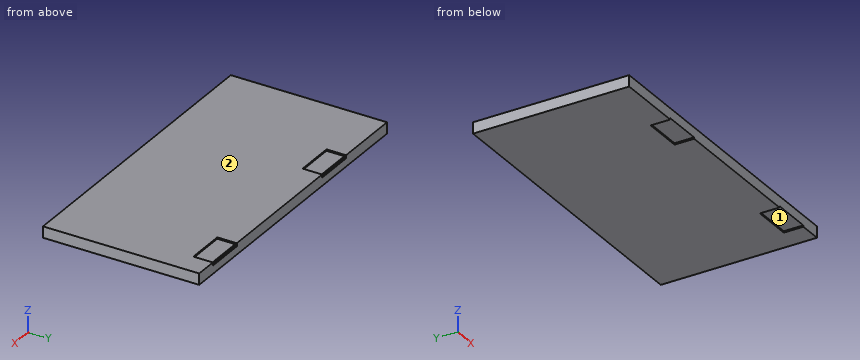
```python
from build123d import *

# Parameters (mm, degrees)
F0_W     = 698.5
F0_H     = 355.6
F1_DEPTH = 25.4
F2_W     = 88.9
F2_H     = 44.45
F3_DEPTH = 3.175
F4_W     = 88.9
F4_H     = 44.45
F5_DEPTH = 3.175
F6_W     = 88.9
F6_H     = 3.81
F7_DEPTH = 3.81
F8_W     = 88.9
F8_H     = 3.81
F9_DEPTH = 3.81


with BuildPart() as f1:
    # F0 (on Top) → F1 (new body)
    with BuildSketch(Plane.XY):
        Rectangle(F0_W, F0_H)
    extrude(amount=F1_DEPTH)

    # F2 (on face) → F3 (cut)
    with BuildSketch(Plane.XY.offset(25.4)):
        with Locations((-152.4, 155.575)):
            Rectangle(F2_W, F2_H)
        with Locations((254, 155.575)):
            Rectangle(F2_W, F2_H)
    extrude(amount=-F3_DEPTH, mode=Mode.SUBTRACT)

    # F4 (on face) → F5 (cut)
    with BuildSketch(Plane(origin=(0, 0, 0), x_dir=(1, 0, 0), z_dir=(0, 0, -1))):
        with Locations((254, 155.575)):
            Rectangle(F4_W, F4_H)
        with Locations((-152.4, 155.575)):
            Rectangle(F4_W, F4_H)
    extrude(amount=-F5_DEPTH, mode=Mode.SUBTRACT)

    # F6 (on face) → F7 (cut)
    with BuildSketch(Plane.XY.offset(22.225)):
        with Locations((-152.4, 175.895)):
            Rectangle(F6_W, F6_H)
    extrude(amount=-F7_DEPTH, mode=Mode.SUBTRACT)

    # F8 (on face) → F9 (cut)
    with BuildSketch(Plane.XY.offset(22.225)):
        with Locations((254, 175.895)):
            Rectangle(F8_W, F8_H)
    extrude(amount=-F9_DEPTH, mode=Mode.SUBTRACT)


solid = f1.part
```
Geometry: final body of the model. Coordinates: model frame, mm. Face numbers are marked on the shaded views. A direction names the side the tool comes from. Give positions to 0.01 mm unless a question says otherwise; leave off trailing zeros. Loops run counter-clockwise (first coordinate to the right, second up) from the corner with the lowest first, then second, coordinate; pieces in that order, holes last. Notation, with made-up numbers: (-9.75, -6) - (4.25, -6) arc R22 cw to (4.25, 20) - close; hole circle Ø2 at (27, 5.5). An arc over 180 degrees is marked (long way). Answer as CSV lines item,"result". Start each with the question number.
(1) Reachability of the marked faces 1 and 2 from +Z, -Z, +X, -X, +Y, -Y: full face, straight path, thin tool, end or side. Return the list, or none.
(2) Section query A-A (x = -166.5). Output: boundary loops of the cut face in (y, z) (3 decimals).
(3) Pin query (flat end, axial travel): P1, Ø3.5, axis at x = 275.5, z = 23, coming from the +Y side; P2, Ø1.1, axis at x = 243.5, y = 176.5, coming from the +Z side (3 decimals); P3, Ø13.5, axis at x = -158, y = -166.5, coming from the -Z side (3 decimals). Return the tip coordinate at first contact, or that it passes through.
(4) Section query B-B (y = -146.5). Output: boundary loops of the cut face in (x, z) (3 decimals).
Worked answers:
1,face 1,"-Z, -Y"
1,face 2,"+Z, +X, -X, +Y, -Y"
2,outline,"(-177.8, 3.175) - (-133.35, 3.175) - (-133.35, 0) - (177.8, 0) - (177.8, 18.415) - (173.99, 18.415) - (173.99, 22.225) - (133.35, 22.225) - (133.35, 25.4) - (-177.8, 25.4) - close"
3,P1,"stops at y = 173.99"
3,P2,"stops at z = 18.415"
3,P3,"stops at z = 3.175"
4,outline,"(-349.25, 0) - (-196.85, 0) - (-196.85, 3.175) - (-107.95, 3.175) - (-107.95, 0) - (209.55, 0) - (209.55, 3.175) - (298.45, 3.175) - (298.45, 0) - (349.25, 0) - (349.25, 25.4) - (-349.25, 25.4) - close"
